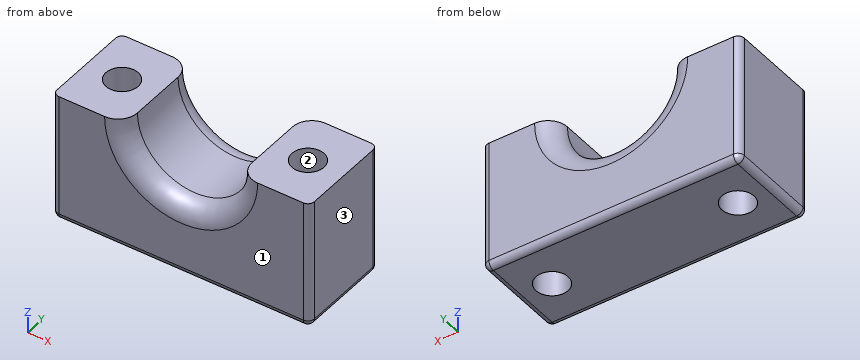
```python
from build123d import *

# Parameters (mm, degrees)
SKETCH_1_W          = 40
SKETCH_1_H          = 40
EXTRUDE_1_DEPTH     = 15
SKETCH_3_R          = 8.9
CUT_EXTRUDE_1_DEPTH = 59.523499554
SKETCH_5_R          = 2.5
CUT_EXTRUDE_2_DEPTH = 59.523499554
SKETCH_6_W          = 40
SKETCH_6_H          = 20
CUT_EXTRUDE_3_DEPTH = 59.523499554
FILLET_1_R          = 3
FILLET_2_R          = 1
FILLET_3_R          = 1
FILLET_4_R          = 1


with BuildPart() as part:
    # 草圖1 → 填料-伸長1 (new body)
    with BuildSketch(Plane(origin=(0, 0, 0), x_dir=(1, 0, 0), z_dir=(0, 1, 0))):
        with Locations((20, 20)):
            Rectangle(SKETCH_1_W, SKETCH_1_H)
    extrude(amount=EXTRUDE_1_DEPTH)

    # 草圖3 → 除料-伸長1 (cut, through all)
    with BuildSketch(Plane(origin=(0, 15, 0), x_dir=(1, 0, 0), z_dir=(0, 1, 0))):
        with Locations(Location((20, 20, 0), (0, 0, 270))):
            Circle(SKETCH_3_R)
    extrude(amount=-CUT_EXTRUDE_1_DEPTH, mode=Mode.SUBTRACT)

    # 草圖5 → 除料-伸長2 (cut, through all)
    with BuildSketch(Plane.XY):
        with Locations((34.45, 7.5)):
            Circle(SKETCH_5_R)
        with Locations(Location((5.55, 7.5, 0), (0, 0, 180))):
            Circle(SKETCH_5_R)
    extrude(amount=-CUT_EXTRUDE_2_DEPTH, mode=Mode.SUBTRACT)

    # 草圖6 → 除料-伸長3 (cut, through all)
    with BuildSketch(Plane(origin=(0, 15, 0), x_dir=(1, 0, 0), z_dir=(0, 1, 0))):
        with Locations((20, 10)):
            Rectangle(SKETCH_6_W, SKETCH_6_H)
    extrude(amount=-CUT_EXTRUDE_3_DEPTH, mode=Mode.SUBTRACT)

    # 圓角1
    fillet_1_edges = [part.edges().sort_by_distance(p)[0] for p in [
        (20, 0, -28.9),
        (20, 15, -28.9),
    ]]
    fillet(fillet_1_edges, radius=FILLET_1_R)

    # 圓角2
    fillet_2_edges = [part.edges().sort_by_distance(p)[0] for p in [
        (20, 15, -40),
        (40, 15, -30),
        (0, 15, -30),
    ]]
    fillet(fillet_2_edges, radius=FILLET_2_R)

    # 圓角3
    # the kernel refuses this fillet: 1 mm, written as the material it takes off along each edge
    with BuildSketch(Plane(origin=(39, 14, -39), x_dir=(0, 0, -1), z_dir=(1, 0, 0))) as fillet_3_piece_1_section:
        Polygon((0, 0), (FILLET_3_R, 0), (FILLET_3_R, FILLET_3_R), (0, FILLET_3_R), align=None)
    fillet_3_piece_1 = extrude(amount=FILLET_3_R, mode=Mode.PRIVATE)
    fillet_3_piece_1 = fillet_3_piece_1 - Plane(origin=(39, 14, -39), x_dir=(0, -0.7071067811865475, 0.7071067811865475), z_dir=(1, 0, 0)) * Sphere(FILLET_3_R, mode=Mode.PRIVATE)
    add(fillet_3_piece_1, mode=Mode.SUBTRACT)
    with BuildSketch(Plane(origin=(1, 14, -39), x_dir=(-1, 0, 0), z_dir=(0, 0, -1))) as fillet_3_piece_2_section:
        Polygon((0, 0), (FILLET_3_R, 0), (FILLET_3_R, FILLET_3_R), (0, FILLET_3_R), align=None)
    fillet_3_piece_2 = extrude(amount=FILLET_3_R, mode=Mode.PRIVATE)
    fillet_3_piece_2 = fillet_3_piece_2 - Plane(origin=(1, 14, -39), x_dir=(0.7071067811865475, -0.7071067811865475, 0), z_dir=(0, 0, -1)) * Sphere(FILLET_3_R, mode=Mode.PRIVATE)
    add(fillet_3_piece_2, mode=Mode.SUBTRACT)
    with BuildSketch(Plane(origin=(0, -2.5, -40), x_dir=(1, 0, 0), z_dir=(0, 1, 0)), Plane(origin=(40, -2.5, -40), x_dir=(0, 0, 1), z_dir=(0, 1, 0))) as fillet_3_piece_3:
        with BuildLine():
            CenterArc((FILLET_3_R, -FILLET_3_R), FILLET_3_R, 90, 90)
            Line((0, -FILLET_3_R), (0, 0))
            Line((0, 0), (FILLET_3_R, 0))
        make_face()
    extrude(amount=16.5, mode=Mode.SUBTRACT)

    # 圓角4
    fillet_4_edges = [part.edges().sort_by_distance(p)[0] for p in [
        (40, 0, -29.5),
        (20, 0, -40),
        (0, 0, -29.5),
        (0.292893219, 0, -39.707106781),
        (39.707106781, 0, -39.707106781),
    ]]
    fillet(fillet_4_edges, radius=FILLET_4_R)


solid = part.part
```
Input: part model. Units: mm. Frame: model coordinates. Face numbers are marked on the shaded views. Round coordinates to 2 decimals unless told otherwise and drop trailing zeros. Loops run counter-clockwise (first coordinate to the right, second up) from the corner with the lowest first, then second, coordinate; pieces in that order, holes last.
1) Section query A-A on x = 34.45. Return the cut outline in (y, z).
Ans:
outline: (0, -39) arc R1 ccw to (1, -40) - (5, -40) - (5, -20) - (0, -20) - close; (10, -40) - (14, -40) arc R1 ccw to (15, -39) - (15, -20) - (10, -20) - close
2) Pin query (flat end, axial travel): pin 1 (4 mm diameter, centred on x = 5.55, y = 7.5, fed in from +Z); pin 2 (6 mm diameter, centred on x = 18, z = -29, fed in from +Y). Return the tip coordinate at first contact, or that it passes through.
Ans:
pin 1: passes through
pin 2: stops at y = 15
3) Material intervals for line 1 (Y direction, x = 5.55, z = -29.25); line 2 (X direction, y = 9.25, z = -33); line 3 (X direction, y = 1, z = -27), sorted ascending.
Ans:
line 1: y = 0 to 5, 10 to 15
line 2: x = 0 to 3.76, 7.34 to 32.66, 36.24 to 40
line 3: x = 0 to 13.34, 26.66 to 40
4) Pull-direction query (Y, two-part tool) for the marked faces 1, 2 and 3; classes: released by +Y, released by -Y, zero draft, split by the parting line, or undercut.
Ans:
face 1: released by -Y
face 2: undercut
face 3: zero draft
5) Section query B-B on y = 7.5. Return the cut outline in (x, z).
Ans:
outline: (0, -39) arc R1 ccw to (1, -40) - (3.05, -40) - (3.05, -20) - (0, -20) - close; (8.05, -40) - (31.95, -40) - (31.95, -20) - (28.9, -20) arc R8.9 cw to (11.1, -20) - (8.05, -20) - close; (36.95, -40) - (39, -40) arc R1 ccw to (40, -39) - (40, -20) - (36.95, -20) - close
6) Section query D-D on x = 20. Return the cut outline in (y, z), plus the area to 3 significant figures.
Ans:
outline: (0, -39) arc R1 ccw to (1, -40) - (14, -40) arc R1 ccw to (15, -39) - (15, -31.9) arc R3 ccw to (12, -28.9) - (3, -28.9) arc R3 ccw to (0, -31.9) - close
area: 162 mm2
7) Section query C-C on z = -38.5. Return the cut outline in (x, y).
Ans:
outline: (0, 1) arc R1 ccw to (1, 0) - (39, 0) arc R1 ccw to (40, 1) - (40, 14) arc R1 ccw to (39, 15) - (1, 15) arc R1 ccw to (0, 14) - close; hole circle Ø5 at (5.55, 7.5); hole circle Ø5 at (34.45, 7.5)
